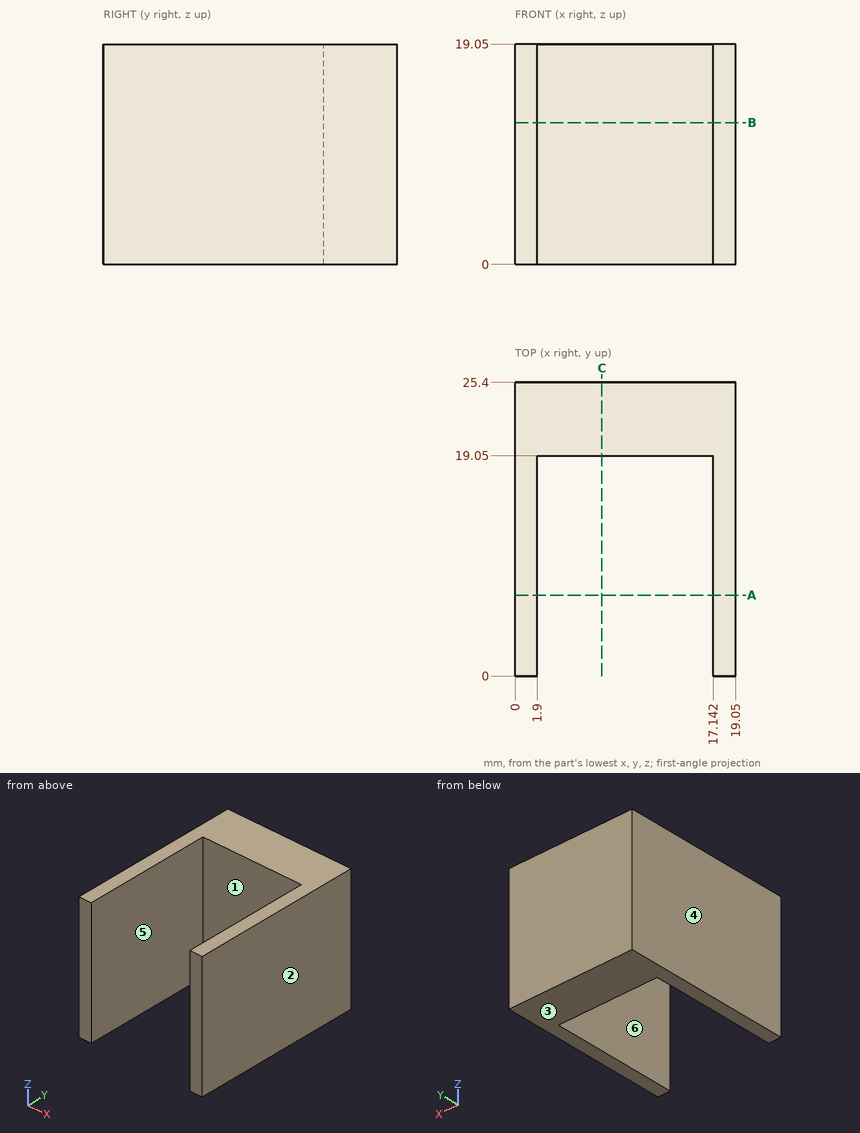
Geometry check sheet. Reference: drawing and pictorial views, mm from the part's lowest x, y, z. A direction names the side the tool comes from. Give positions to 0.01 mm unless a question says otherwise; leave off trailing zeros. Order: outer loops, then holes, each group sorted by start corner. A loop starts at its lowest first (then second) coordinate and runs counter-clockwise, first axis right, second up. Notation, with made-up numbers: M 86,-25 L 121,-25 A17 cw 121,-1 Z; hole C 21,81.25 d3. An arc over 180 degrees is marked long. Use one line per item in the form item = value. Start each with the question number.
Q1. Section check A-A (y = 7). Enter the section's corners in (x, z).
Q2. Section check B-B (z = 12.25). Enter the section's corners in (x, y).
Q3. Mould release check, pull along X, two halves, no side actions. Record for the marked faces 3, 4, 5 and 6: +X half, -X half, draft (parallel to the pull), parting line (faces both ways), or undercut.
Q4. Access from +Z, -Z, +X, -X, +Y, -Y to the whole of each face (thin tool, end or side, straight path). Record for the marked faces 1 and 2.
Q5. Go/stop test with a flat-tipped pin: pin 1 Ø3 at (x, z) = (6, 15) entering from -Y. Record where the tip stops, or that it passes through.
Q6. Section check C-C (x = 7.5). Enter the section's corners in (y, z).
Q7. Scan lines: line 1 along X through (y, z) = (16.5, 13.25); line 2 along Y through (x, z) = (15.5, 18). Record each from-to range of solid material in increasing order. Write a range as [from, to].
Evaluation:
q1.outline = M 0,0 L 1.9,0 L 1.9,19.05 L 0,19.05 Z; M 17.14,0 L 19.05,0 L 19.05,19.05 L 17.14,19.05 Z
q2.outline = M 0,0 L 1.9,0 L 1.9,19.05 L 17.14,19.05 L 17.14,0 L 19.05,0 L 19.05,25.4 L 0,25.4 Z
q3.face_3 = draft
q3.face_4 = -X half
q3.face_5 = undercut
q3.face_6 = undercut
q4.face_1 = +Z, -Z, -Y
q4.face_2 = +Z, -Z, +X, +Y, -Y
q5.pin_1 = 19.05
q6.outline = M 19.05,0 L 25.4,0 L 25.4,19.05 L 19.05,19.05 Z
q7.line_1 = [0, 1.9], [17.14, 19.05]
q7.line_2 = [19.05, 25.4]
